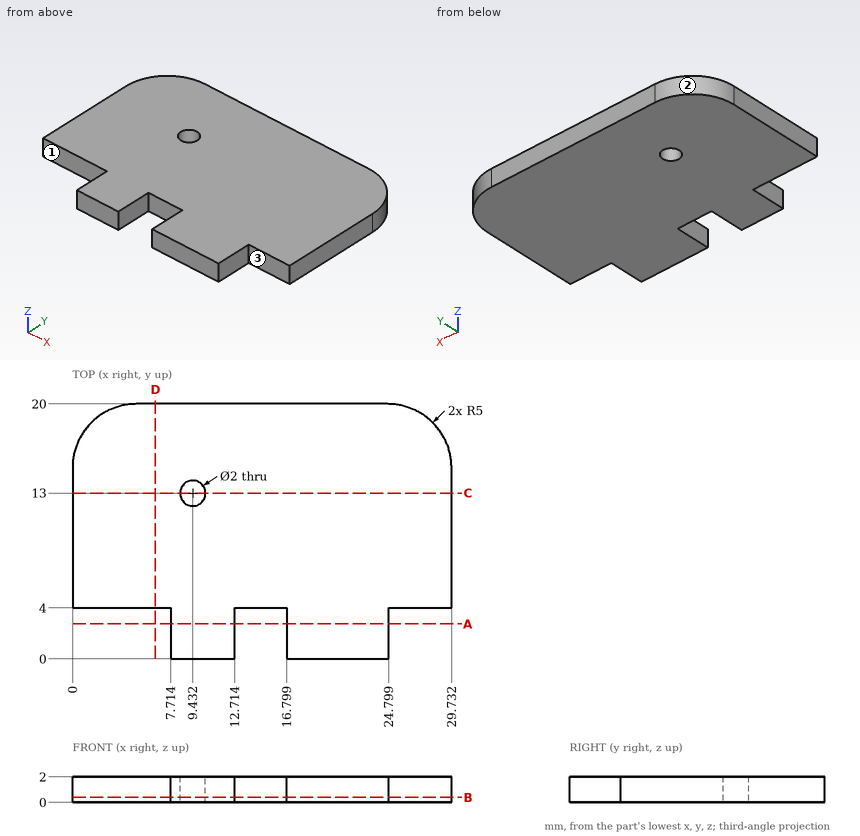
Input: dimensioned drawing with shaded views. Units: mm. Origin: part minimum x, y, z. A direction names the side the tool comes from. Coordinates: 2 decimals unless noted, no trailing zeros. Write each loop counter-clockwise with the first axis right and the second up, starting at its lowest first coordinate (ties: lowest second). Pieces come first, ordered by that corner, then holes. Notation, with made-up numbers: M 47.25,-24 L 53.25,-24 A21 ccw 53.25,2 Z; hole C -29,-7 d10. An arc over 180 degrees is marked long. Answer as CSV lines item,"result". Start each with the question number.
Q1. Cut plane A-A on y = 2.75. Return the cut outline in (x, z).
Q2. Line query: line 1 (X direction, y = 15.25, z = 0.4) (1 decimal); line 2 (Y direction, x = 8.75, z = 0.75); line 3 (Y direction, x = 15.5, z = 0.45). Output: solid intervals per line, ascending. Write a range as from..to.
Q3. Pin query (flat end, axial travel): P1, Ø1, axis at x = 25.5, z = 1, coming from the +Y side; P2, Ø1, axis at y = 2.5, z = 1.5, coming from the +X side; P3, Ø0.6, axis at x = 5.5, z = 0.5, coming from the -Y side. Return the tip coordinate at first contact, or that it passes through.
Q4. Cut plane B-B on z = 0.4. Return the cut outline in (x, y).
Q5. Cut plane C-C on y = 13. Return the cut outline in (x, z).
Q6. Cut plane D-D on x = 6.5. Return the cut outline in (y, z).
Q7. Reachability of the marked faces 1, 2 and 3 from +Z, -Z, +X, -X, +Y, -Y: full face, straight path, thin tool, end or side. Return the list, or none.
Findings below:
1,outline,"M 7.71,0 L 12.71,0 L 12.71,2 L 7.71,2 Z; M 16.8,0 L 24.8,0 L 24.8,2 L 16.8,2 Z"
2,line 1,"x = 0..29.7"
2,line 2,"y = 0..12.27, 13.73..20"
2,line 3,"y = 4..20"
3,P1,"stops at y = 19.99"
3,P2,"stops at x = 24.8"
3,P3,"stops at y = 4"
4,outline,"M 0,4 L 7.71,4 L 7.71,0 L 12.71,0 L 12.71,4 L 16.8,4 L 16.8,0 L 24.8,0 L 24.8,4 L 29.73,4 L 29.73,15 A5 ccw 24.73,20 L 5,20 A5 ccw 0,15 Z; hole C 9.43,13 d2"
5,outline,"M 0,0 L 8.43,0 L 8.43,2 L 0,2 Z; M 10.43,0 L 29.73,0 L 29.73,2 L 10.43,2 Z"
6,outline,"M 4,0 L 20,0 L 20,2 L 4,2 Z"
7,face 1,"+Z, -Z, -X, -Y"
7,face 2,"+Z, -Z, -X, +Y"
7,face 3,"+Z, -Z, +X, -Y"
